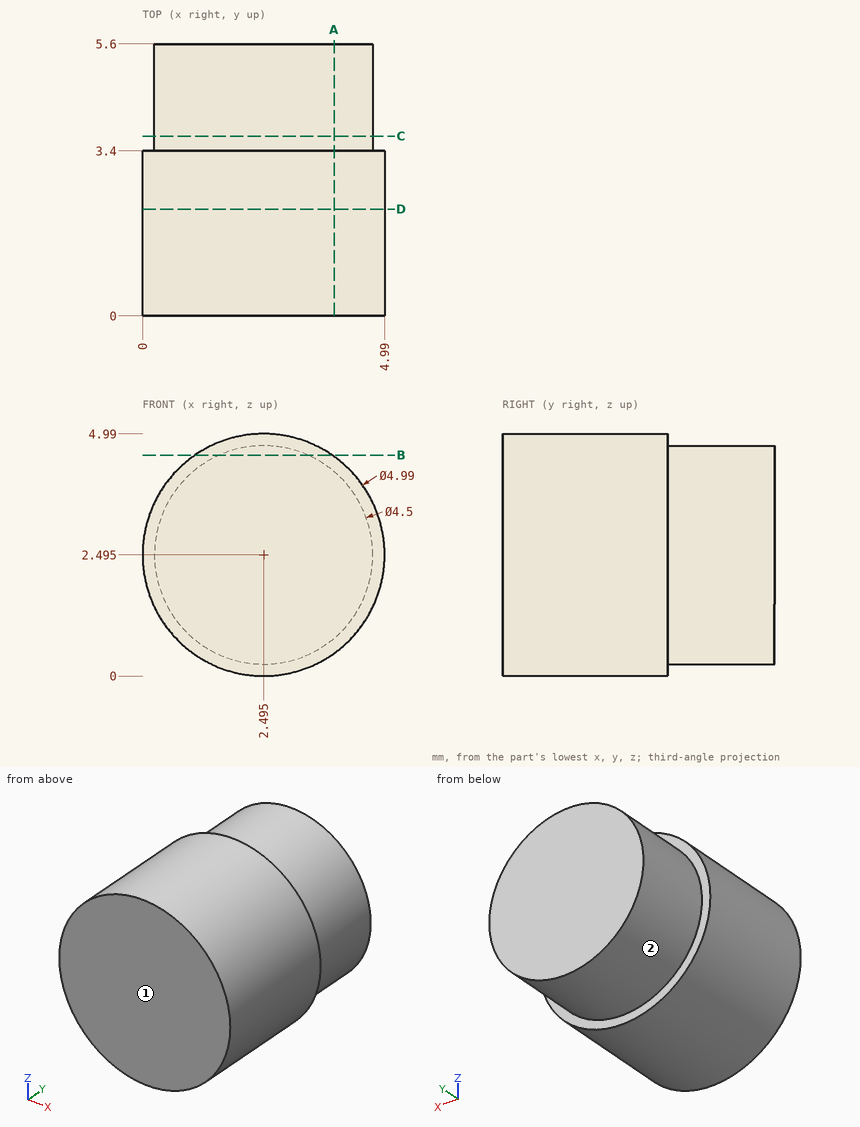
For this review, use the dimensioned drawing (mm, ordinates from the lowest corner) and the shaded views. A direction names the side the tool comes from. Round coordinates to 2 decimals unless told otherwise and drop trailing zeros. Order: outer loops, then holes, each group sorted by start corner. A loop starts at its lowest first (then second) coordinate and runs counter-clockwise, first axis right, second up. Notation, with made-up numbers: M 79,45.25 L 89,45.25 A38 ccw 89,84.25 Z; hole C 79,25.5 d6. An arc over 180 degrees is marked long. Use a Markdown table: item, result. Add a question column.
Item 1: Tool access review of the marked faces 1 and 2: name each direction out of +Z, -Z, +X, -X, +Y, -Y from which nothing blocks a thin tool from reaching the whole face with its end or side.
Item 2: Add section C-C, the plane y = 3.7. Give the boundary of the cut face in (x, z) (3 decimals), then the cut area to 3 significant figures.
Item 3: To check wall thickness, follow line 1 along Y through (x, z) = (4.45, 1); line 2 along Z through (x, y) = (2.6, 2.7); line 3 along X through (y, z) = (2.35, 3.35). State the ranges of each line that lie inside material, in increasing order.
Item 4: Add section A-A, the plane x = 3.95. Give the boundary of the cut face in (y, z), then the cut area to 3 significant figures.
Item 5: Add section D-D, the plane y = 2.2. Give the boundary of the cut face in (x, z) (3 decimals), then the cut area to 3 significant figures.
Item 6: Insertion check: pin 1 (1 mm diameter, centred on y = 2.5, z = 1.5, fed in from -X); pin 2 (1.5 mm diameter, centred on y = 3, z = 4, fed in from -X). Each pin has a flat end and moves straight along its axis. Give the tip position at first contact, or say it passes through.
Item 7: Add section B-B, the plane z = 4.55. Give the boundary of the cut face in (x, y), then the cut area to 3 significant figures.
Geometry results:
| question | item | result |
|---|---|---|
| 1 | face 1 | +Z, -Z, +X, -X, -Y |
| 1 | face 2 | +Y |
| 2 | outline | C 2.495,2.495 d4.5 |
| 2 | area | 15.9 mm² |
| 3 | line 1 | y = 0 to 3.4 |
| 3 | line 2 | z = 0 to 4.99 |
| 3 | line 3 | x = 0.15 to 4.84 |
| 4 | outline | M 0,0.47 L 3.4,0.47 L 3.4,0.78 L 5.6,0.78 L 5.6,4.21 L 3.4,4.21 L 3.4,4.52 L 0,4.52 Z |
| 4 | area | 21.3 mm² |
| 5 | outline | C 2.495,2.495 d4.99 |
| 5 | area | 19.6 mm² |
| 6 | pin 1 | stops at x = 0.05 |
| 6 | pin 2 | stops at x = 0.12 |
| 7 | outline | M 1.08,0 L 3.91,0 L 3.91,3.4 L 3.41,3.4 L 3.41,5.6 L 1.58,5.6 L 1.58,3.4 L 1.08,3.4 Z |
| 7 | area | 13.7 mm² |
